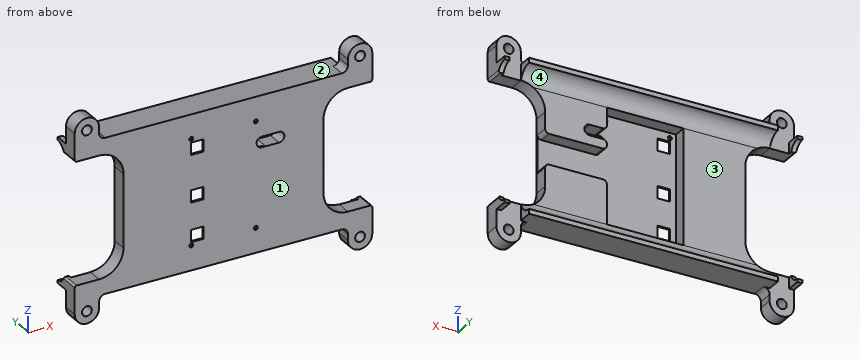
from build123d import *

# Parameters (mm, degrees)
BOSS_EXTRUDE1_DEPTH         = 7.9375
F_10_CLEARANCE_HOLE1_D      = 5.1054
SKETCH8_W                   = 2.54
SKETCH8_H                   = 1.5875
SKETCH8_W_2                 = 129.68
SKETCH8_H_2                 = 2.54
BOSS_EXTRUDE2_DEPTH         = 7.5
SKETCH10_W                  = 2.54
SKETCH10_H                  = 71.825
BOSS_EXTRUDE3_DEPTH         = 1.5875
FILLET3_R                   = 3.175
FILLET4_R                   = 5.9125
FILLET5_R                   = 7.5
SKETCH11_W                  = 25.4
SKETCH11_H                  = 63.5
CUT_EXTRUDE1_DEPTH          = 96.03828495
FILLET6_R                   = 12.7
SKETCH12_W                  = 40
SKETCH12_H                  = 60
CUT_EXTRUDE2_DEPTH          = 6.9375
SKETCH13_W                  = 57.54
SKETCH13_H                  = 15.8
CUT_EXTRUDE3_DEPTH          = 6.9375
CUT_EXTRUDE4_DEPTH          = 95.111439835
SKETCH15_W                  = 6.35
SKETCH15_H                  = 6.35
CUT_EXTRUDE5_DEPTH          = 95.880981267
FILLET7_R                   = 2.032
F_45_0_082_DIAMETER_HOLE1_D = 2.0828
FILLET8_R                   = 1.016


with BuildPart() as part:
    # Sketch1 → Boss-Extrude1 (new body)
    with BuildSketch(Plane(origin=(0, 0, 0), x_dir=(1, 0, 0), z_dir=(0, 1, 0))):
        with BuildLine():
            Line((77.54, -40.04), (77.54, 40.04))
            Line((77.54, 40.04), (77.54, 46.39))
            ThreePointArc((77.54, 46.39), (71.19, 52.74), (64.84, 46.39))
            Line((64.84, 46.39), (64.84, 40.04))
            Line((64.84, 40.04), (-64.84, 40.04))
            Line((-64.84, 40.04), (-64.84, 46.39))
            ThreePointArc((-64.84, 46.39), (-71.19, 52.74), (-77.54, 46.39))
            Line((-77.54, 46.39), (-77.54, 40.04))
            Line((-77.54, 40.04), (-77.54, -40.04))
            Line((-77.54, -40.04), (-77.54, -46.39))
            ThreePointArc((-77.54, -46.39), (-71.19, -52.74), (-64.84, -46.39))
            Line((-64.84, -46.39), (-64.84, -40.04))
            Line((-64.84, -40.04), (64.84, -40.04))
            Line((64.84, -40.04), (64.84, -46.39))
            ThreePointArc((64.84, -46.39), (71.19, -52.74), (77.54, -46.39))
            Line((77.54, -46.39), (77.54, -40.04))
        make_face()
    extrude(amount=BOSS_EXTRUDE1_DEPTH)

    # #10 Clearance Hole1 (through all)
    with Locations(Plane(origin=(0, 7.9375, 0), x_dir=(1, 0, 0), z_dir=(0, 1, 0))):
        with Locations((-71.19, 46.39), (71.19, 46.39), (71.19, -46.39), (-71.19, -46.39)):
            Hole(F_10_CLEARANCE_HOLE1_D / 2)

    # Sketch8 → Boss-Extrude2 (add)
    with BuildSketch(Plane(origin=(0, 7.9375, 0), x_dir=(1, 0, 0), z_dir=(0, 1, 0))):
        with Locations((-76.27, 36.70625)):
            Rectangle(SKETCH8_W, SKETCH8_H)
        with Locations((76.27, 36.70625)):
            Rectangle(SKETCH8_W, SKETCH8_H)
        with Locations((76.27, -36.70625)):
            Rectangle(SKETCH8_W, SKETCH8_H)
        with Locations((-76.27, -36.70625)):
            Rectangle(SKETCH8_W, SKETCH8_H)
        with Locations((0, 38.77)):
            Rectangle(SKETCH8_W_2, SKETCH8_H_2)
        with Locations((0, -38.77)):
            Rectangle(SKETCH8_W_2, SKETCH8_H_2)
    extrude(amount=BOSS_EXTRUDE2_DEPTH)

    # Sketch10 → Boss-Extrude3 (add)
    with BuildSketch(Plane(origin=(0, 7.9375, 0), x_dir=(1, 0, 0), z_dir=(0, 1, 0))):
        with Locations((-76.27, 0)):
            Rectangle(SKETCH10_W, SKETCH10_H)
        with Locations((76.27, 0)):
            Rectangle(SKETCH10_W, SKETCH10_H)
    extrude(amount=BOSS_EXTRUDE3_DEPTH)

    # Fillet3
    fillet3_edges = [part.edges().sort_by_distance(p)[0] for p in [
        (64.84, 3.96875, 40.04),
        (-64.84, 3.96875, 40.04),
        (-64.84, 3.96875, -40.04),
        (64.84, 3.96875, -40.04),
    ]]
    fillet(fillet3_edges, radius=FILLET3_R)

    # Fillet4
    fillet4_edges = [part.edges().sort_by_distance(p)[0] for p in [
        (76.27, 9.525, 35.9125),
        (76.27, 9.525, -35.9125),
        (-76.27, 9.525, 35.9125),
        (-76.27, 9.525, -35.9125),
    ]]
    fillet(fillet4_edges, radius=FILLET4_R - 0.0001)  # a hair under: the kernel refuses the full size

    # Fillet5
    fillet5_edges = [part.edges().sort_by_distance(p)[0] for p in [
        (0, 7.9375, 37.5),
        (0, 7.9375, -37.5),
    ]]
    fillet(fillet5_edges, radius=FILLET5_R - 0.0001)  # a hair under: the kernel refuses the full size

    # Sketch11 → Cut-Extrude1 (cut, through all)
    with BuildSketch(Plane.XZ):
        with Locations((-64.84, 0)):
            Rectangle(SKETCH11_W, SKETCH11_H)
        with Locations((64.84, 0)):
            Rectangle(SKETCH11_W, SKETCH11_H)
    extrude(amount=-CUT_EXTRUDE1_DEPTH, mode=Mode.SUBTRACT)

    # Fillet6
    fillet6_edges = [part.edges().sort_by_distance(p)[0] for p in [
        (-52.14, 4.072251385, 31.75),
    ]]
    fillet(fillet6_edges, radius=FILLET6_R)
    fillet6_2_edges = [part.edges().sort_by_distance(p)[0] for p in [
        (-52.14, 4.072251385, -31.75),
    ]]
    fillet(fillet6_2_edges, radius=FILLET6_R)
    fillet6_3_edges = [part.edges().sort_by_distance(p)[0] for p in [
        (52.14, 4.072251385, -31.75),
    ]]
    fillet(fillet6_3_edges, radius=FILLET6_R)
    fillet6_4_edges = [part.edges().sort_by_distance(p)[0] for p in [
        (52.14, 4.072251385, 31.75),
    ]]
    fillet(fillet6_4_edges, radius=FILLET6_R)

    # Sketch12 → Cut-Extrude2 (cut)
    with BuildSketch(Plane(origin=(0, 7.9375, 0), x_dir=(1, 0, 0), z_dir=(0, 1, 0))):
        Rectangle(SKETCH12_W, SKETCH12_H)
    extrude(amount=-CUT_EXTRUDE2_DEPTH, mode=Mode.SUBTRACT)

    # Sketch13 → Cut-Extrude3 (cut)
    with BuildSketch(Plane(origin=(0, 7.9375, 0), x_dir=(1, 0, 0), z_dir=(0, 1, 0))):
        with Locations((48.77, -0.5)):
            Rectangle(SKETCH13_W, SKETCH13_H)
    extrude(amount=-CUT_EXTRUDE3_DEPTH, mode=Mode.SUBTRACT)

    # Sketch14 → Cut-Extrude4 (cut, through all)
    with BuildSketch(Plane(origin=(0, 7.9375, 0), x_dir=(1, 0, 0), z_dir=(0, 1, 0))):
        with BuildLine():
            Line((29, -18.78), (20, -18.78))
            ThreePointArc((20, -18.78), (17.25, -16.03), (20, -13.28))
            Line((20, -13.28), (29, -13.28))
            ThreePointArc((29, -13.28), (31.75, -16.03), (29, -18.78))
        make_face()
    extrude(amount=-CUT_EXTRUDE4_DEPTH, mode=Mode.SUBTRACT)

    # Sketch15 → Cut-Extrude5 (cut, through all)
    with BuildSketch(Plane(origin=(0, 1, 0), x_dir=(1, 0, 0), z_dir=(0, 1, 0))):
        with Locations((-13.65, 2.06)):
            Rectangle(SKETCH15_W, SKETCH15_H)
        with Locations((-13.65, 22.38)):
            Rectangle(SKETCH15_W, SKETCH15_H)
        with Locations((-13.65, -22.38)):
            Rectangle(SKETCH15_W, SKETCH15_H)
    extrude(amount=-CUT_EXTRUDE5_DEPTH, mode=Mode.SUBTRACT)

    # Fillet7
    fillet7_edges = [part.edges().sort_by_distance(p)[0] for p in [
        (52.14, 4.46875, -7.4),
        (20, 4.46875, -7.4),
        (52.14, 4.46875, 8.4),
        (20, 4.46875, 8.4),
        (20, 4.46875, 18.78),
        (20, 4.46875, 13.28),
    ]]
    fillet(fillet7_edges, radius=FILLET7_R)

    # #45 (0.082) Diameter Hole1 (through all)
    with Locations(Plane(origin=(0, 1, 0), x_dir=(1, 0, 0), z_dir=(0, 1, 0))):
        with Locations((-16.825, 27.206), (16.825, -27.46), (-16.825, -27.46), (16.825, 27.206)):
            Hole(F_45_0_082_DIAMETER_HOLE1_D / 2)

    # Fillet8
    fillet8_edges = [part.edges().sort_by_distance(p)[0] for p in [
        (-77.54, 4.894947012, -31.75),
        (-77.54, 4.894947012, 31.75),
        (77.54, 4.894947012, 31.75),
        (77.54, 4.894947012, -31.75),
    ]]
    fillet(fillet8_edges, radius=FILLET8_R)


solid = part.part
Can you work these out from the model? Positions are in its coordinate system, mm. Face numbers are marked on the shaded views. A direction names the side the tool comes from. Give positions to 0.01 mm unless a question says otherwise; leave off trailing zeros. Write each loop counter-clockwise with the first axis right and the second up, starting at its lowest first coordinate (ties: lowest second). Pieces come first, ordered by that corner, then holes. Notation, with made-up numbers: M 49.5,-14 L 75.5,-14 A29 cw 75.5,11 Z; hole C -10,9.25 d5. An arc over 180 degrees is marked long. Answer in a Markdown table with one row per item. Add a question column.
Item 1: Imagine slicing it at D-D, the plane z = -12. Write out the boundary of the cut face in (x, y), plus the area to 3 significant figures.
Item 2: Imagine slicing it at B-B, the plane x = -71.19. Write out the boundary of the cut face in (y, z).
Item 3: For pin 1 Ø6 at (y, z) = (10.5, 5.5) entering from -X; pin 2 Ø5.5 at (x, y) = (41, 5) entering from +Z; pin 3 Ø4.5 at (y, z) = (13, 33.5) entering from +X; pin 4 Ø3.5 at (y, z) = (4.5, 27.5) entering from -X, each with a flat end and sliding along its axis, tell me the tip position at first contact or that it passes through.
Item 4: Imagine slicing it at A-A, the plane y = 13.75. Write out the boundary of the cut face in (x, z), plus the area to 3 significant figures.
Item 5: We'd pull the mould along X, two halves only. Please class the marked faces 1 and 2: released by +X, released by -X, zero draft, split by the parting line, or undercut.
Item 6: Please list where these lines run through material, in increasing order: L1, parallel to Z at x = -71.19, y = 5.75; L2, parallel to X at y = 5.5, z = -46.39; L3, parallel to X at y = 2, z = -19.5.
Item 7: On a 3-axis mill with a long thin cutter (end or side, diameter ignored), from which of +Z, -Z, +X, -X, +Y, -Y can I reach the whole of each face in a straight line? I mean the marked faces 3 and 4. Say none if no direction works.
Evaluation:
| question | item | result |
|---|---|---|
| 1 | outline | M -52.14,0 L 52.14,0 L 52.14,7.94 L 20,7.94 L 20,1 L -20,1 L -20,7.94 L -52.14,7.94 Z |
| 1 | area | 550 mm² |
| 2 | outline | M 0,-52.74 L 7.94,-52.74 L 7.94,-48.94 L 0,-48.94 Z; M 0,-43.84 L 7.94,-43.84 L 7.94,-31.75 L 0,-31.75 Z; M 0,31.75 L 7.94,31.75 L 7.94,43.84 L 0,43.84 Z; M 0,48.94 L 7.94,48.94 L 7.94,52.74 L 0,52.74 Z |
| 3 | pin 1 | stops at x = -52.14 |
| 3 | pin 2 | stops at z = 40.04 |
| 3 | pin 3 | stops at x = 77.54 |
| 3 | pin 4 | stops at x = -57.27 |
| 4 | outline | M -77.54,-37.5 L -75,-37.5 L -75,-35.67 L -77.54,-35.67 Z; M -77.54,35.67 L -75,35.67 L -75,37.5 L -77.54,37.5 Z; M -64.84,-40.04 L 64.84,-40.04 L 64.84,-37.31 L -64.84,-37.31 Z; M -64.84,37.31 L 64.84,37.31 L 64.84,40.04 L -64.84,40.04 Z; M 75,-37.5 L 77.54,-37.5 L 77.54,-35.67 L 75,-35.67 Z; M 75,35.67 L 77.54,35.67 L 77.54,37.5 L 75,37.5 Z |
| 4 | area | 727 mm² |
| 5 | face 1 | zero draft |
| 5 | face 2 | undercut |
| 6 | L1 | z = -52.74 to -48.94, -43.84 to -31.75, 31.75 to 43.84, 48.94 to 52.74 |
| 6 | L2 | x = -77.54 to -73.74, -68.64 to -64.84, 64.84 to 68.64, 73.74 to 77.54 |
| 6 | L3 | x = -52.15 to -20, 20 to 52.15 |
| 7 | face 3 | +X, -X, +Y |
| 7 | face 4 | +Y |
